The listing builds one solid part. Answer for the finished solid, in the listing's coordinates (mm). Give positions to 0.01 mm unless a question says otherwise; leave off trailing zeros. Write each loop counter-clockwise with the first axis right and the second up, starting at its lowest first coordinate (ties: lowest second). Pieces come first, ordered by that corner, then holes. Notation, with made-up numbers: M -10.5,74.5 L 29.5,74.5 A28 cw 29.5,98.5 Z; hole C 73,20 d4. An arc over 180 degrees is marked long. Return JSON: item names as keys, results as strings.
from build123d import *

# Parameters (mm, degrees)
SKETCH2_W           = 52
SKETCH2_H           = 2.6
BOSS_EXTRUDE1_DEPTH = 2.5


with BuildPart() as part:
    # Sketch2 → Boss-Extrude1 (new body)
    with BuildSketch(Plane(origin=(0, 0, 0), x_dir=(1, 0, 0), z_dir=(0, 1, 0))):
        Polygon((35, 25), (35, 77.6), (-35, 77.6), (-35, 25), (-39, 25), (-39, -25), (-35, -25), (-35, -47.6), (-15, -47.6), (-15, -67.6), (-35, -67.6), (-35, -77.6), (35, -77.6), (35, -25), (39, -25), (39, 25), align=None)
        with Locations((0, 73.3)):
            Rectangle(SKETCH2_W, SKETCH2_H, mode=Mode.SUBTRACT)
        with Locations((0, -73.3)):
            Rectangle(SKETCH2_W, SKETCH2_H, mode=Mode.SUBTRACT)
    extrude(amount=BOSS_EXTRUDE1_DEPTH)


solid = part.part
Item 1: A cutting plane is placed at A-A, the plane x = -20.5. Write down the section's boundary in (y, z), plus the area to 3 significant figures.
Geometry results:
{"outline": "M 0,-77.6 L 2.5,-77.6 L 2.5,-74.6 L 0,-74.6 Z; M 0,-72 L 2.5,-72 L 2.5,47.6 L 0,47.6 Z; M 0,67.6 L 2.5,67.6 L 2.5,72 L 0,72 Z; M 0,74.6 L 2.5,74.6 L 2.5,77.6 L 0,77.6 Z", "area": "325 mm2"}
Item 2: Given pin 1 Ø1.2 at (y, z) = (1.5, 40) entering from +X; pin 2 Ø1.2 at (x, y) = (-37.5, 1.5) entering from +Z; pin 3 Ø0.8 at (y, z) = (1, 32) entering from -X, each flat-ended and moving along its own axis, determine where each tip first touches the part or whether it passes through.
Geometry results:
{"pin 1": "stops at x = 35", "pin 2": "stops at z = 25", "pin 3": "stops at x = -35"}
Item 3: A cutting plane is placed at B-B, the plane y = 2.1. Write down the section's boundary in (x, z), plus the area to 3 significant figures.
Geometry results:
{"outline": "M -39,-25 L -35,-25 L -35,-77.6 L 35,-77.6 L 35,-25 L 39,-25 L 39,25 L 35,25 L 35,77.6 L -35,77.6 L -35,67.6 L -15,67.6 L -15,47.6 L -35,47.6 L -35,25 L -39,25 Z; hole M -26,-74.6 L 26,-74.6 L 26,-72 L -26,-72 Z; hole M -26,72 L 26,72 L 26,74.6 L -26,74.6 Z", "area": "10,600 mm2"}
Item 4: Determine the mould class of faces 1 (the flat face through (-1, 2.5, -1)), 2 (the flat face through (-1, 0, -1)) for opening direction Y: +Y half, -Y half, draft (parallel to the pull), parting line (faces both ways), or undercut.
Geometry results:
{"face 1": "+Y half", "face 2": "-Y half"}
Item 5: A cutting plane is placed at D-D, the plane z = 29. Write down the section's boundary in (x, y), plus the area to 3 significant figures.
Geometry results:
{"outline": "M -35,0 L 35,0 L 35,2.5 L -35,2.5 Z", "area": "175 mm2"}
Item 6: Find the intervals of material crossed by line 1 (Z direction, x = 13, y = 0.8); line 2 (Z direction, x = -20.5, y = 0.55); line 3 (Z direction, x = -32, y = 0.9), in increasing order.
Geometry results:
{"line 1": "z = -77.6 to -74.6, -72 to 72, 74.6 to 77.6", "line 2": "z = -77.6 to -74.6, -72 to 47.6, 67.6 to 72, 74.6 to 77.6", "line 3": "z = -77.6 to 47.6, 67.6 to 77.6"}
Item 7: A cutting plane is placed at C-C, the plane x = -10.5. Write down the section's boundary in (y, z).
Geometry results:
{"outline": "M 0,-77.6 L 2.5,-77.6 L 2.5,-74.6 L 0,-74.6 Z; M 0,-72 L 2.5,-72 L 2.5,72 L 0,72 Z; M 0,74.6 L 2.5,74.6 L 2.5,77.6 L 0,77.6 Z"}
